Source: CAD feature listing. Evaluate the final solid. Frame: model axes, mm. Face numbers are marked on the shaded views. Coordinates: 2 decimals unless noted, no trailing zeros. Write each loop counter-clockwise with the first axis right and the second up, starting at its lowest first coordinate (ties: lowest second). Pieces come first, ordered by that corner, then holes. Notation, with made-up numbers: (-30.5, 79) - (1.5, 79) arc R19 cw to (1.5, 92) - close; hole circle Ø3 at (-30, -19.5). An arc over 180 degrees is marked (long way). One line per item, written item: value.
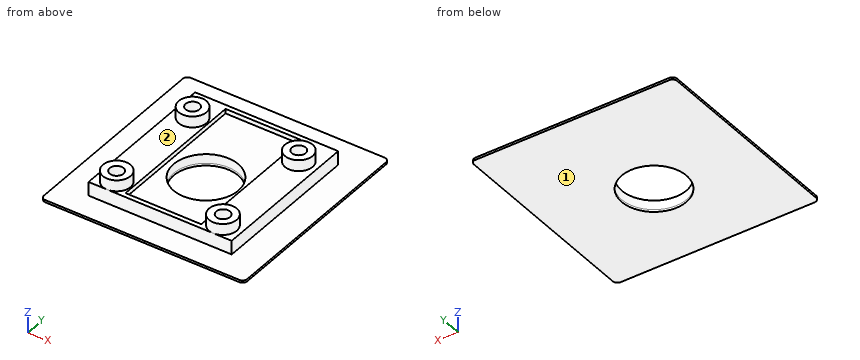
from build123d import *

# Parameters (mm, degrees)
F0_W      = 31
F0_H      = 33
F1_DEPTH  = 2
F2_R      = 3
F3_DEPTH  = 2.4
F4_W      = 16.4
F4_H      = 31
F5_DEPTH  = 1
F6_R      = 1.5
F7_DEPTH  = 3.4
F8_R      = 1.5
F9_DEPTH  = 3.4
F10_R     = 7
F11_DEPTH = 25
F12_DEPTH = 1
F13_W     = 44
F13_H     = 45
F13_W_2   = 31
F13_H_2   = 33
F13_R     = 7
F14_DEPTH = 0.5
F15_R     = 1


with BuildPart() as f1:
    # F0 (on Top) → F1 (new body)
    with BuildSketch(Plane.XY):
        with Locations((15.5, 16.5)):
            Rectangle(F0_W, F0_H)
    extrude(amount=F1_DEPTH)

    # F2 (on face) → F3 (join)
    with BuildSketch(Plane.XY.offset(2)):
        with Locations((4, 3)):
            Circle(F2_R)
        with Locations((4, 26.5)):
            Circle(F2_R)
        with Locations((27, 26.5)):
            Circle(F2_R)
        with Locations((27, 3)):
            Circle(F2_R)
    extrude(amount=F3_DEPTH)

    # F4 (on face) → F5 (cut)
    with BuildSketch(Plane.XY.offset(2)):
        with Locations((15.5, 16.5)):
            Rectangle(F4_W, F4_H)
    extrude(amount=-F5_DEPTH, mode=Mode.SUBTRACT)

    # F6 (on face) → F7 (cut)
    with BuildSketch(Plane.XY.offset(4.4)):
        with Locations((27, 26.5)):
            Circle(F6_R)
    extrude(amount=-F7_DEPTH, mode=Mode.SUBTRACT)

    # F8 (on face) → F9 (cut)
    with BuildSketch(Plane.XY.offset(4.4)):
        with Locations((4, 26.5)):
            Circle(F8_R)
        with Locations((4.0643862449, 2.8885749634)):
            Circle(F8_R)
        with Locations((27.0567759871, 3.0037942342)):
            Circle(F8_R)
    extrude(amount=-F9_DEPTH, mode=Mode.SUBTRACT)

    # F10 (on face) → F11 (cut)
    with BuildSketch(Plane.XY.offset(1)):
        with Locations((15.5, 14.2)):
            Circle(F10_R)
    extrude(amount=-F11_DEPTH, mode=Mode.SUBTRACT)

    # F12 (add): a face of the model
    f12_faces = [f1.faces().sort_by_distance(p)[0] for p in [
        (0.4527692569, 16.5, 0),
    ]]
    extrude(f12_faces, amount=F12_DEPTH)

    # F13 (on face) → F14 (join)
    with BuildSketch(Plane(origin=(0, 0, -1), x_dir=(1, 0, 0), z_dir=(0, 0, -1))):
        with Locations((15.5, -17)):
            Rectangle(F13_W, F13_H)
        with Locations((15.5, -16.5)):
            Rectangle(F13_W_2, F13_H_2, mode=Mode.SUBTRACT)
        with Locations((15.5, -16.5)):
            Rectangle(F13_W_2, F13_H_2)
        with Locations((15.5, -14.2)):
            Circle(F13_R, mode=Mode.SUBTRACT)
    extrude(amount=F14_DEPTH)

    # F15
    f15_edges = [f1.edges().sort_by_distance(p)[0] for p in [
        (-6.5, -5.5, -1.25),
        (37.5, -5.5, -1.25),
        (37.5, 39.5, -1.25),
        (-6.5, 39.5, -1.25),
    ]]
    fillet(f15_edges, radius=F15_R)


solid = f1.part
1) Draft query along Y for the marked faces 1 and 2. Return one class per face: released by +Y, released by -Y, zero draft, split by the parting line, or undercut.
Values found:
face 1: zero draft
face 2: undercut
2) Material intervals for line 1 (Y direction, x = 27, z = 2.7); line 2 (Y direction, x = 4, z = 2.6); line 3 (Y direction, x = 15.5, z = -1.3), sorted ascending.
Values found:
line 1: 0 to 1.5, 4.5 to 6, 23.5 to 25, 28 to 29.5
line 2: 0 to 1.39, 4.39 to 6, 23.5 to 25, 28 to 29.5
line 3: -5.5 to 7.2, 21.2 to 39.5
3) Section query B-B on z = 3.4. Output: boundary loops of the cut face in (x, y), then the cut area to 3 significant figures.
Values found:
outline: circle Ø6 at (4, 3); circle Ø6 at (4, 26.5); circle Ø6 at (27, 3); circle Ø6 at (27, 26.5); hole circle Ø3 at (4, 26.5); hole circle Ø3 at (4.06, 2.89); hole circle Ø3 at (27, 26.5); hole circle Ø3 at (27.06, 3)
area: 84.8 mm2
4) Section query D-D on y = 26.5. Output: boundary loops of the cut face in (x, z).
Values found:
outline: (-6.5, -1.5) - (37.5, -1.5) - (37.5, -1) - (31, -1) - (31, 2) - (30, 2) - (30, 4.4) - (28.5, 4.4) - (28.5, 1) - (25.5, 1) - (25.5, 4.4) - (24, 4.4) - (24, 2) - (23.7, 2) - (23.7, 1) - (7.3, 1) - (7.3, 2) - (7, 2) - (7, 4.4) - (5.5, 4.4) - (5.5, 1) - (2.5, 1) - (2.5, 4.4) - (1, 4.4) - (1, 2) - (0, 2) - (0, -1) - (-6.5, -1) - close
5) Section query A-A on y = 14.2. Output: boundary loops of the cut face in (x, z), then the cut area to 3 significant figures.
Values found:
outline: (-6.5, -1.5) - (8.5, -1.5) - (8.5, 1) - (7.3, 1) - (7.3, 2) - (0, 2) - (0, -1) - (-6.5, -1) - close; (22.5, -1.5) - (37.5, -1.5) - (37.5, -1) - (31, -1) - (31, 2) - (23.7, 2) - (23.7, 1) - (22.5, 1) - close
area: 63.6 mm2
6) Section query C-C on x = 15.5. Output: boundary loops of the cut face in (y, z), then the cut area to 3 significant figures.
Values found:
outline: (-5.5, -1.5) - (7.2, -1.5) - (7.2, 1) - (1, 1) - (1, 2) - (0, 2) - (0, -1) - (-5.5, -1) - close; (21.2, -1.5) - (39.5, -1.5) - (39.5, -1) - (33, -1) - (33, 2) - (32, 2) - (32, 1) - (21.2, 1) - close
area: 55.5 mm2
7) Contact query for flat-ended pins moving along their axis: P1, Ø3, axis at y = 2.5, z = 4, coming from the -X side; P2, Ø2.5, axis at x = 27.5, y = 27, coming from the +Z side; P3, Ø10, axis at x = -1, y = 11.5, coming from the +Z side; P4, Ø0.9, axis at x = 4, y = 2.5, coming from the +Z side. Output: stop coordinate, or through.
Values found:
P1: x = 1
P2: z = 4.4
P3: z = 2
P4: z = 1
